from build123d import *

# Parameters (mm, degrees)
EXTRUDE_1_DEPTH = 20


with BuildPart() as part:
    # 草图1 → 凸台-拉伸1 (new body)
    with BuildSketch(Plane.XY):
        with BuildLine():
            Line((56.568542495, 20), (123.431457505, 20))
            ThreePointArc((123.431457505, 20), (140.098124172, 22.859547921), (154.858425558, 31.111111111))
            ThreePointArc((154.858425558, 31.111111111), (220, 0), (154.858425558, -31.111111111))
            ThreePointArc((154.858425558, -31.111111111), (140.098124172, -22.859547921), (123.431457505, -20))
            Line((123.431457505, -20), (56.568542495, -20))
            ThreePointArc((56.568542495, -20), (39.901875828, -22.859547921), (25.141574442, -31.111111111))
            ThreePointArc((25.141574442, -31.111111111), (-40, 0), (25.141574442, 31.111111111))
            ThreePointArc((25.141574442, 31.111111111), (39.901875828, 22.859547921), (56.568542495, 20))
        make_face()
    extrude(amount=EXTRUDE_1_DEPTH)


solid = part.part
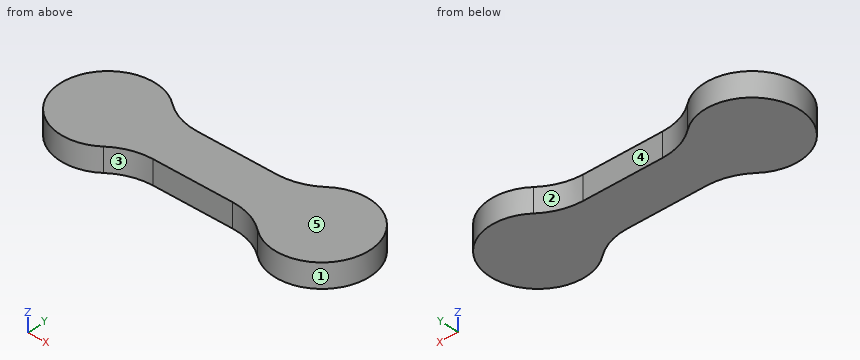
Can you work these out from the model? Positions are in its coordinate system, mm. Face numbers are marked on the shaded views. A direction names the side the tool comes from. Round coordinates to 2 decimals unless told otherwise and drop trailing zeros. Loops run counter-clockwise (first coordinate to the right, second up) from the corner with the lowest first, then second, coordinate; pieces in that order, holes last. Notation, with made-up numbers: (51, 21) - (79, 21) arc R30 cw to (79, 55) - close; hole circle Ø3 at (14, 24.25). An arc over 180 degrees is marked (long way). Answer in a Markdown table with one row per item. Add a question column.
Q1. Which directions (+Z, -Z, +X, -X, +Y, -Y) give clear straight access to the entire face, cutting with the end or side of a thin tool? Please do the marked faces 1, 2 and 3.
Q2. For pin 1 Ø4 at (x, z) = (193.5, 8) entering from -Y; pin 2 Ø5 at (y, z) = (17, 7.5) entering from -X; pin 3 Ø1.5 at (y, z) = (-9.5, 12) entering from -X; pin 4 Ø5 at (x, y) = (123, 21) entering from +Z, each with a flat end and sliding along its axis, tell me the tip position at first contact or that it passes through.
Q3. I want a section at C-C on x = 137. List the corners of the cut face in (y, z) for me, and give its area (3 significant figures).
Q4. I want a section at A-A on z = 3. List the corners of the cut face in (x, y) for me, and give its area (3 significant figures).
Q5. We'd pull the mould along X, two halves only. Please class the marked faces 4 and 5: pulls with the +X half, pulls with the -X half, needs draft (parallel to the pull), parting line crosses it, or undercut.
Q6. I need wall thicknesses on L1, parallel to X at y = -35.5, z = 12.5; L2, parallel to X at y = -24, z = 13.5; L3, parallel to Y at x = 123, z = 16. Which ranges of each line are inside material? Lowest first, please.
Q7. I want a section at B-B on x = 65.5. List the corners of the cut face in (y, z) for me, and give its area (3 significant figures).
A:
| question | item | result |
|---|---|---|
| 1 | face 1 | +Z, -Z |
| 1 | face 2 | +Z, -Z, +Y |
| 1 | face 3 | +Z, -Z, -Y |
| 2 | pin 1 | y = -38.31 |
| 2 | pin 2 | x = -37.28 |
| 2 | pin 3 | x = -39.03 |
| 2 | pin 4 | z = 20 |
| 3 | outline | (-21.88, 0) - (21.88, 0) - (21.88, 20) - (-21.88, 20) - close |
| 3 | area | 875 mm^2 |
| 4 | outline | (25.14, -31.11) arc R50 cw to (56.57, -20) - (123.43, -20) arc R50 cw to (154.86, -31.11) arc R40 ccw (long way) to (154.86, 31.11) arc R50 cw to (123.43, 20) - (56.57, 20) arc R50 cw to (25.14, 31.11) arc R40 ccw (long way) to start |
| 4 | area | 14,400 mm^2 |
| 5 | face 4 | undercut |
| 5 | face 5 | needs draft |
| 6 | L1 | -18.43 to 18.43, 161.57 to 198.43 |
| 6 | L2 | -32 to 36.97, 143.03 to 212 |
| 6 | L3 | -20 to 20 |
| 7 | outline | (-20, 0) - (20, 0) - (20, 20) - (-20, 20) - close |
| 7 | area | 800 mm^2 |
